Autodesk Inventor part; units mm, degrees
ref_plane "YZ Plane" through (0, 0, 0) normal (1, 0, 0) x (0, 1, 0)
ref_plane "XZ Plane" through (0, 0, 0) normal (0, 1, 0) x (-1, 0, 0)
ref_plane "XY Plane" through (0, 0, 0) normal (0, 0, 1) x (1, 0, 0)
sketch "草圖1" plane through (0, 0, 0) normal (1, 0, 0) x (0, 1, 0)
  circle A0 centre (0, 0) radius 2.5
  circle A1 centre (0, 0) radius 15
  dimension "d0" = 5
  dimension "d1" = 30
extrude "擠出1" add sketch "草圖1" along normal mid plane 3
sketch "草圖2" plane through (1.5, 0, 0) normal (1, 0, 0) x (0, 0, -1)
  line L0 (-9.5551, 8.1555) -> (8.9449, 8.1555)
  line L1 (8.9449, 8.1555) -> (8.9449, 5.1555)
  line L2 (8.9449, 5.1555) -> (-9.5551, 5.1555)
  line L3 (-9.5551, 5.1555) -> (-9.5551, 8.1555)
  point P0 (0, 0)
  dimension "d4" = 18.5
  dimension "d5" = 3
extrude "擠出2" add sketch "草圖2" along normal blind 47
sketch "草圖3" plane through (1.5, 8.1555, 9.5551) normal (0, 1, 0) x (1, 0, 0)
  line L0 (0, 18.5) -> (47, 18.5) construction
  line L1 (41, 18.5) -> (17, 18.5)
  line L2 (17, 18.5) -> (17, 6)
  line L3 (17, 6) -> (41, 6)
  line L4 (41, 6) -> (41, 18.5)
  line L5 (47, 18.5) -> (47, 0) construction
  line L6 (47, 0) -> (47, 18.5)
  line L7 (47, 12.25) -> (14.3759, 12.25) construction
  circle A0 centre (43.5, 12.25) radius 1.25
  line L8 (29, 12.25) -> (29, 6) construction
  circle A1 centre (14.5, 12.25) radius 1.25
  point P0 (-1.5, 9.5551)
  point P1 (41, 12.25)
  dimension "d8" = 24
  dimension "d9" = 12.5
  dimension "d10" = 6
  dimension "d11" = 2.5
  dimension "d12" = 29
extrude "擠出3" cut sketch "草圖3" against normal up to surface (3 mm away)
sketch "草圖4" plane through (1.5, 0, 0) normal (1, 0, 0) x (0, 0, -1)
  line L0 (-9.5551, 8.1555) -> (8.9449, 8.1555)
  line L1 (-12.5892, 8.1555) -> (12.5892, 8.1555)
  circle A0 centre (0, 0) radius 15
extrude "擠出4" cut sketch "草圖4" against normal up to surface (3 mm away) contours L1 A0 L0 picked at (-0.2034, 10.437)
properties part number "Arm_2"
Input: part model. Units: mm. Frame: model coordinates. A direction names the side the tool comes from. Round coordinates to 2 decimals unless told otherwise and drop trailing zeros. Order: outer loops, then holes, each group sorted by start corner. A loop starts at its lowest first (then second) coordinate and runs counter-clockwise, first axis right, second up. Notation, with made-up numbers: (16, 73) - (20, 73) arc R22 cw to (20, 104) - close; hole circle Ø3 at (33, 31.25). An arc over 180 degrees is marked (long way). Answer as a JSON object with one key per item and string values. Group by question number.
(1) Cut plane A-A (y = 0). Return loops of the section in (x, z).
(2) Reachability of faces 1 (the face through (25, 7, 9.555)), 2 (the face through (19, 5.156, 4)), 3 (the face through (10, 7, -8.945)) from +Z, -Z, +X, -X, +Y, -Y: full face, straight path, thin tool, end or side. Return the list, or none.
(3) Cut plane C-C (x = 45). Return loops of the section in (y, z), then the cut area to 3 significant figures.
(4) Material intervals for probe 1 along Z at (x, y) = (0.3, 0); probe 2 along X at (y, z) = (7, 2.5); probe 3 along Z at (x, y) = (16, 7.4), sorted ascending. Write a range as from..to.
(5) Pin query (flat end, axial travel): P1, Ø6, axis at x = 5.5, z = -4, coming from the -Y side; P2, Ø0.9, axis at x = 9, y = 6, coming from the -Z side; P3, Ø0.9, axis at x = 36, y = 7, coming from the +Z side. Return the tip coordinate at first contact, or that it passes through.
(6) Cut plane B-B (z = 0). Return loops of the section in (x, y).
(7) Cut plane D-D (z = 9). Return loops of the section in (x, y), then the cut area to 3 significant figures.
(8) Draft query along X for faces 4 (the face through (48.5, 7, 0)), 5 (the face through (45, 7, -8.945)), 6 (the face through (-1.5, -4, 0)), 7 (the face through (30, 7, 3.555)). Return one class per face: released by +X, released by -X, zero draft, split by the parting line, or undercut.
Here are the results:
{
 "1": {"outline": "(-1.5, -15) - (1.5, -15) - (1.5, -2.5) - (-1.5, -2.5) - close; (-1.5, 2.5) - (1.5, 2.5) - (1.5, 15) - (-1.5, 15) - close"},
 "2": {"face 1": "+Z, +X, +Y, -Y", "face 2": "+Z, -Z, +X, -Y", "face 3": "-Z, +X, +Y, -Y"},
 "3": {"outline": "(5.16, -8.94) - (8.16, -8.94) - (8.16, -3.94) - (5.16, -3.94) - close; (5.16, -1.44) - (8.16, -1.44) - (8.16, 9.56) - (5.16, 9.56) - close", "area": "48.0 mm^2"},
 "4": {"probe 1": "z = -15..-2.5, 2.5..15", "probe 2": "x = -1.5..18.5, 42.5..48.5", "probe 3": "z = -8.94..-3.94, -1.44..9.56"},
 "5": {"P1": "stops at y = 5.16", "P2": "stops at z = -8.94", "P3": "stops at z = 9.56"},
 "6": {"outline": "(-1.5, -15) - (1.5, -15) - (1.5, -2.5) - (-1.5, -2.5) - close; (-1.5, 2.5) - (1.5, 2.5) - (1.5, 5.16) - (18.5, 5.16) - (18.5, 8.16) - (-1.5, 8.16) - close; (42.5, 5.16) - (48.5, 5.16) - (48.5, 8.16) - (42.5, 8.16) - close"},
 "7": {"outline": "(-1.5, -12) - (1.5, -12) - (1.5, 5.16) - (48.5, 5.16) - (48.5, 8.16) - (-1.5, 8.16) - close", "area": "201 mm^2"},
 "8": {"face 4": "released by +X", "face 5": "zero draft", "face 6": "released by -X", "face 7": "undercut"}
}
